```python
from build123d import *

# Parameters (mm, degrees)
SKETCH1_W             = 184.6
SKETCH1_H             = 106.1
BOSS_EXTRUDE1_DEPTH   = 10
CUT_EXTRUDE2_REACH    = 110.92
SKETCH7_R             = 1.7
SKETCH3_W             = 164.6
SKETCH3_H             = 10
BOSS_EXTRUDE2_DEPTH   = 21.625
FILLET1_R             = 10
SKETCH5_R             = 1.7
BOSS_EXTRUDE3_DEPTH   = 10
SKETCH6_R             = 5
CUT_EXTRUDE1_DEPTH    = 4
FILLET2_R             = 10
FILLET2_OF_MIRROR1_R  = 10
MIRROR2_START         = 84.6
MIRROR2_OUTLINE_R     = 5
MIRROR2_DEPTH         = 10
MIRROR2_2_OUTLINE_R   = 5
MIRROR2_2_OUTLINE_R_2 = 1.7
MIRROR2_2_DEPTH       = 6


# Read off the part's stored shape, not the designer's step: Mirror2
with BuildPart() as part:
    # Sketch1 → Boss-Extrude1 (new body)
    with BuildSketch(Plane.XY):
        with Locations((2.3, 0)):
            Rectangle(SKETCH1_W, SKETCH1_H)
    extrude(amount=BOSS_EXTRUDE1_DEPTH)

    # Sketch7 → Cut-Extrude2 (cut, up to next)
    with BuildSketch(Plane(origin=(0, 0, 0), x_dir=(-1, 0, 0), z_dir=(0, 0, -1)), mode=Mode.PRIVATE) as cut_extrude2_sk1:
        with Locations((-10, 0)):
            Circle(SKETCH7_R)
    cut_extrude2_tool1 = extrude(cut_extrude2_sk1.sketch, amount=-CUT_EXTRUDE2_REACH, mode=Mode.PRIVATE) & part.part
    # Sketch7 → Cut-Extrude2 (cut, up to next)
    with BuildSketch(Plane(origin=(0, 0, 0), x_dir=(-1, 0, 0), z_dir=(0, 0, -1)), mode=Mode.PRIVATE) as cut_extrude2_sk2:
        with Locations((-5, 8.660254038)):
            Circle(SKETCH7_R)
    cut_extrude2_tool2 = extrude(cut_extrude2_sk2.sketch, amount=-CUT_EXTRUDE2_REACH, mode=Mode.PRIVATE) & part.part
    # Sketch7 → Cut-Extrude2 (cut, up to next)
    with BuildSketch(Plane(origin=(0, 0, 0), x_dir=(-1, 0, 0), z_dir=(0, 0, -1)), mode=Mode.PRIVATE) as cut_extrude2_sk3:
        with Locations((5, 8.660254038)):
            Circle(SKETCH7_R)
    cut_extrude2_tool3 = extrude(cut_extrude2_sk3.sketch, amount=-CUT_EXTRUDE2_REACH, mode=Mode.PRIVATE) & part.part
    # Sketch7 → Cut-Extrude2 (cut, up to next)
    with BuildSketch(Plane(origin=(0, 0, 0), x_dir=(-1, 0, 0), z_dir=(0, 0, -1)), mode=Mode.PRIVATE) as cut_extrude2_sk4:
        with Locations((10, 0)):
            Circle(SKETCH7_R)
    cut_extrude2_tool4 = extrude(cut_extrude2_sk4.sketch, amount=-CUT_EXTRUDE2_REACH, mode=Mode.PRIVATE) & part.part
    # Sketch7 → Cut-Extrude2 (cut, up to next)
    with BuildSketch(Plane(origin=(0, 0, 0), x_dir=(-1, 0, 0), z_dir=(0, 0, -1)), mode=Mode.PRIVATE) as cut_extrude2_sk5:
        with Locations((5, -8.660254038)):
            Circle(SKETCH7_R)
    cut_extrude2_tool5 = extrude(cut_extrude2_sk5.sketch, amount=-CUT_EXTRUDE2_REACH, mode=Mode.PRIVATE) & part.part
    # Sketch7 → Cut-Extrude2 (cut, up to next)
    with BuildSketch(Plane(origin=(0, 0, 0), x_dir=(-1, 0, 0), z_dir=(0, 0, -1)), mode=Mode.PRIVATE) as cut_extrude2_sk6:
        with Locations((-5, -8.660254038)):
            Circle(SKETCH7_R)
    cut_extrude2_tool6 = extrude(cut_extrude2_sk6.sketch, amount=-CUT_EXTRUDE2_REACH, mode=Mode.PRIVATE) & part.part
    add(cut_extrude2_tool1.solids().sort_by_distance((10, 0, 0))[0], mode=Mode.SUBTRACT)
    add(cut_extrude2_tool2.solids().sort_by_distance((5, 8.660254, 0))[0], mode=Mode.SUBTRACT)
    add(cut_extrude2_tool3.solids().sort_by_distance((-5, 8.660254, 0))[0], mode=Mode.SUBTRACT)
    add(cut_extrude2_tool4.solids().sort_by_distance((-10, 0, 0))[0], mode=Mode.SUBTRACT)
    add(cut_extrude2_tool5.solids().sort_by_distance((-5, -8.660254, 0))[0], mode=Mode.SUBTRACT)
    add(cut_extrude2_tool6.solids().sort_by_distance((5, -8.660254, 0))[0], mode=Mode.SUBTRACT)

    # Sketch3 → Boss-Extrude2 (add)
    with BuildSketch(Plane.XY.offset(10)):
        with Locations((2.3, 48.05)):
            Rectangle(SKETCH3_W, SKETCH3_H)
        with Locations((2.3, -48.05)):
            Rectangle(SKETCH3_W, SKETCH3_H)
    extrude(amount=BOSS_EXTRUDE2_DEPTH)

    # Fillet1
    fillet1_edges = [part.edges().sort_by_distance(p)[0] for p in [
        (2.3, 43.05, 31.625),
        (2.3, -43.05, 31.625),
    ]]
    fillet(fillet1_edges, radius=FILLET1_R - 0.0001)  # a hair under: the kernel refuses the full size

    # Sketch5 → Boss-Extrude3 (add)
    with BuildSketch(Plane.ZY.offset(80)):
        with BuildLine():
            Line((31.625, 53.05), (31.625, 38))
            ThreePointArc((31.625, 38), (28.870383682, 31.349767926), (22.220151608, 28.595151608))
            Line((22.220151608, 28.595151608), (10, 28.595151608))
            Line((10, 28.595151608), (10, 53.05))
            Line((10, 53.05), (31.625, 53.05))
        make_face()
        with Locations(Location((22.220151608, 38, 0), (0, 0, 270))):
            Circle(SKETCH5_R, mode=Mode.SUBTRACT)
    boss_extrude3 = extrude(amount=BOSS_EXTRUDE3_DEPTH)

    # Sketch6 → Cut-Extrude1 (cut)
    with BuildSketch(Plane.ZY.offset(90)):
        with Locations((22.220151608, 38)):
            Circle(SKETCH6_R)
    cut_extrude1 = extrude(amount=-CUT_EXTRUDE1_DEPTH, mode=Mode.SUBTRACT)

    # Fillet2
    fillet2_edges = [part.edges().sort_by_distance(p)[0] for p in [
        (-85, 28.595151608, 10),
    ]]
    fillet(fillet2_edges, radius=FILLET2_R)

    # Mirror1: Boss-Extrude3, Cut-Extrude1 across plane
    add(boss_extrude3.mirror(Plane.ZX))
    add(cut_extrude1.mirror(Plane.ZX), mode=Mode.SUBTRACT)

    # Fillet2 of Mirror1
    fillet2_of_mirror1_edges = [part.edges().sort_by_distance(p)[0] for p in [
        (-85, -28.595151608, 10),
    ]]
    fillet(fillet2_of_mirror1_edges, radius=FILLET2_OF_MIRROR1_R)

    # Mirror2 outline → Mirror2 (add)
    # profile 1 of 2: a face of its own
    with BuildSketch(Plane.YZ.offset(MIRROR2_START)):
        with BuildLine():
            ThreePointArc((38, 31.625), (31.349767926, 28.870383682), (28.595151608, 22.220151608))
            Line((28.595151608, 22.220151608), (28.595151608, 20))
            ThreePointArc((28.595151608, 20), (25.66621942, 12.928932188), (18.595151608, 10))
            Line((18.595151608, 10), (53.05, 10))
            Line((53.05, 10), (53.05, 31.625))
            Line((53.05, 31.625), (38, 31.625))
        make_face()
        with Locations((38, 22.220151608)):
            Circle(MIRROR2_OUTLINE_R, mode=Mode.SUBTRACT)
    # profile 2 of 2: a face of its own
    with BuildSketch(Plane.YZ.offset(MIRROR2_START)):
        with BuildLine():
            Line((-53.05, 10), (-18.595151608, 10))
            ThreePointArc((-18.595151608, 10), (-25.66621942, 12.928932188), (-28.595151608, 20))
            Line((-28.595151608, 20), (-28.595151608, 22.220151608))
            ThreePointArc((-28.595151608, 22.220151608), (-31.349767926, 28.870383682), (-38, 31.625))
            Line((-38, 31.625), (-53.05, 31.625))
            Line((-53.05, 31.625), (-53.05, 10))
        make_face()
        with Locations((-38, 22.220151608)):
            Circle(MIRROR2_OUTLINE_R, mode=Mode.SUBTRACT)
    extrude(amount=MIRROR2_DEPTH)

    # Mirror2 2 outline → Mirror2 2 (add)
    # profile 1 of 2: a face of its own
    with BuildSketch(Plane.YZ.offset(MIRROR2_START)):
        with Locations((38, 22.220151608)):
            Circle(MIRROR2_2_OUTLINE_R)
        with Locations((38, 22.220151608)):
            Circle(MIRROR2_2_OUTLINE_R_2, mode=Mode.SUBTRACT)
    # profile 2 of 2: a face of its own
    with BuildSketch(Plane.YZ.offset(MIRROR2_START)):
        with Locations((-38, 22.220151608)):
            Circle(MIRROR2_2_OUTLINE_R)
        with Locations((-38, 22.220151608)):
            Circle(MIRROR2_2_OUTLINE_R_2, mode=Mode.SUBTRACT)
    extrude(amount=MIRROR2_2_DEPTH)


solid = part.part
```
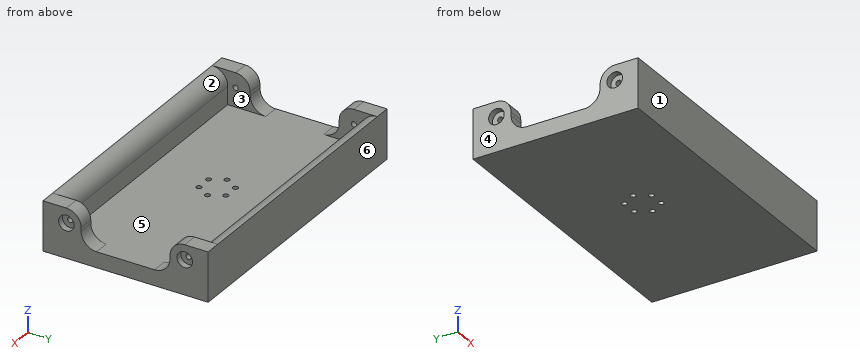
Design review of the part built by this model. Coordinates are the model's own, in mm. Face numbers are marked on the shaded views. A direction names the side the tool comes from. Round coordinates to 2 decimals unless told otherwise and drop trailing zeros. Write each loop counter-clockwise with the first axis right and the second up, starting at its lowest first coordinate (ties: lowest second). Pieces come first, ordered by that corner, then holes.
Item 1: For the marked faces 5 and 6, list the 3-axis set-ups (+Z, -Z, +X, -X, +Y, -Y) from which the entire face can be reached by the end or side of a thin tool; tool diameter is ignored.
Item 2: We need section C-C on y = -46. Write out the cut boundary in (x, z) (3 decimals).
Item 3: The part is to be moulded in two halves that separate along X. For the marked faces 1, 2, 3 and 4, say which applies: +X half, -X half, draft (parallel to the pull), parting line (faces both ways), or undercut.
Item 4: We need section D-D on y = 24. Write out the cut boundary in (x, z).
Item 5: We need section A-A on z = 13.5. Write out the cut boundary in (x, y), and give its area (3 significant figures).
Item 6: For probe 1 along X at (y, z) = (-36, 16); probe 2 along Y at (x, z) = (-37.5, 13.5); probe 3 along X at (y, z) = (-1, 8), list the stretches that pass through material, from the lowest coordinate up.
Item 7: Clearance check with flat-ended pins moving along their axes: pin 1 Ø3 at (y, z) = (-38, 22.22) entering from +X; pin 2 Ø16 at (y, z) = (38, 22.22) entering from +X; pin 3 Ø10 at (x, y) = (-3.5, -22.5) entering from +Z; pin 4 Ø8 at (y, z) = (-38, 22.22) entering from +X. State where each tip first meets the part, or that it passes through.
Returned:
1. face 5: +Z
1. face 6: +Z, -Z, +X, -X, +Y
2. outline: (-90, 0) - (94.6, 0) - (94.6, 31.625) - (84.6, 31.625) - (84.6, 28.717) - (-80, 28.717) - (-80, 31.625) - (-90, 31.625) - close
3. face 1: draft
3. face 2: undercut
3. face 3: undercut
3. face 4: -X half
4. outline: (-90, 0) - (94.6, 0) - (94.6, 11.59) - (84.6, 11.59) - (84.6, 10) - (-80, 10) - (-80, 11.59) - (-90, 11.59) - close
5. outline: (-90, -53.05) - (94.6, -53.05) - (94.6, -26.19) - (84.6, -26.19) - (84.6, -43.05) - (-80, -43.05) - (-80, -26.19) - (-90, -26.19) - close; (-90, 26.19) - (-80, 26.19) - (-80, 43.05) - (84.6, 43.05) - (84.6, 26.19) - (94.6, 26.19) - (94.6, 53.05) - (-90, 53.05) - close
5. area: 4,370 mm2
6. probe 1: x = -90 to -80, 84.6 to 94.6
6. probe 2: y = -53.05 to -43.05, 43.05 to 53.05
6. probe 3: x = -90 to -11.37, -8.63 to 8.63, 11.37 to 94.6
7. pin 1: passes through
7. pin 2: stops at x = 94.6
7. pin 3: stops at z = 10
7. pin 4: stops at x = 90.6
